Here's how the part is built. I have some questions about the finished solid (model axes, mm). Face numbers are marked on the shaded views. A direction names the side the tool comes from. Coordinates: 2 decimals unless noted, no trailing zeros. Order: outer loops, then holes, each group sorted by start corner. A loop starts at its lowest first (then second) coordinate and runs counter-clockwise, first axis right, second up. Notation, with made-up numbers: (-29.5, 79) - (-4.5, 79) arc R18 ccw to (-4.5, 103) - close; hole circle Ø1 at (-23.75, 26). An arc over 180 degrees is marked (long way). Answer in a Markdown table with one row per item. Add a question column.
Item 1: Will these pins go through, and if not, where does the flat tip stop? pin 1 Ø3 at (x, z) = (-2, 8) entering from -Y; pin 2 Ø5.5 at (x, y) = (-2.5, -0.5) entering from +Z; pin 3 Ø5 at (x, z) = (-1.5, 10) entering from -Y; pin 4 Ø2 at (y, z) = (-3.5, 7.5) entering from +X.
Item 2: I want a section at C-C (z = 4.75). Please give me the cut outline in (x, y).
Item 3: If I drill on line 1 along Z through (x, y) = (-4, 2.25); line 2 along Y through (x, z) = (0, 5.5); line 3 along Z through (x, y) = (1.75, 2.25), over which ranges is the centre line in solid material (lowest first)? Write a range as from..to.
Item 4: I want a section at A-A (y = 0). Please give me the cut outline in (x, z).
Item 5: I want a section at B-B (x = 4.5). Please give me the cut outline in (y, z).
Item 6: On a 3-axis mill with a long thin cutter (end or side, diameter ignored), from which of +Z, -Z, +X, -X, +Y, -Y can I reach the whole of each face in a straight line? I mean the marked faces 1 and 2. Say none if no direction works.
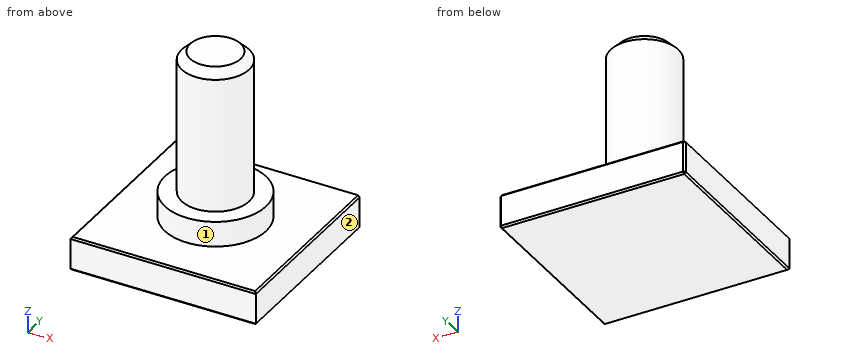
```python
from build123d import *

# Parameters (mm, degrees)
SKETCH1_W           = 11
SKETCH1_H           = 11
BOSS_EXTRUDE1_DEPTH = 2
SKETCH2_R           = 2
BOSS_EXTRUDE2_DEPTH = 10
CHAMFER1_SIZE       = 0.1
SKETCH3_R           = 3
BOSS_EXTRUDE3_DEPTH = 1.5
CHAMFER2_SIZE       = 0.5


with BuildPart() as part:
    # Sketch1 → Boss-Extrude1 (new body)
    with BuildSketch(Plane.XY):
        Rectangle(SKETCH1_W, SKETCH1_H)
    extrude(amount=BOSS_EXTRUDE1_DEPTH)

    # Sketch2 → Boss-Extrude2 (add)
    with BuildSketch(Plane.XY.offset(2)):
        Circle(SKETCH2_R)
    extrude(amount=BOSS_EXTRUDE2_DEPTH)

    # Chamfer1
    chamfer1_edges = [part.edges().sort_by_distance(p)[0] for p in [
        (-5.5, 0, 2),
        (0, -5.5, 2),
        (5.5, 0, 2),
        (0, -5.5, 0),
        (-5.5, 0, 0),
        (0, 5.5, 0),
        (5.5, 0, 0),
        (0, 5.5, 2),
        (-5.5, 5.5, 1),
        (5.5, 5.5, 1),
    ]]
    chamfer(chamfer1_edges, length=CHAMFER1_SIZE)

    # Sketch3 → Boss-Extrude3 (add)
    with BuildSketch(Plane.XY.offset(2)):
        Circle(SKETCH3_R)
    extrude(amount=BOSS_EXTRUDE3_DEPTH)

    # Chamfer2
    chamfer2_edges = [part.edges().sort_by_distance(p)[0] for p in [
        (-2, 0, 12),
    ]]
    chamfer(chamfer2_edges, length=CHAMFER2_SIZE)


solid = part.part
```
Values follow:
| question | item | result |
|---|---|---|
| 1 | pin 1 | stops at y = -1.94 |
| 1 | pin 2 | stops at z = 12 |
| 1 | pin 3 | stops at y = -2 |
| 1 | pin 4 | passes through |
| 2 | outline | circle Ø4 at (0, 0) |
| 3 | line 1 | z = 0..2 |
| 3 | line 2 | y = -2..2 |
| 3 | line 3 | z = 0..3.5 |
| 4 | outline | (-5.5, 0.1) - (-5.4, 0) - (5.4, 0) - (5.5, 0.1) - (5.5, 1.9) - (5.4, 2) - (3, 2) - (3, 3.5) - (2, 3.5) - (2, 11.5) - (1.5, 12) - (-1.5, 12) - (-2, 11.5) - (-2, 3.5) - (-3, 3.5) - (-3, 2) - (-5.4, 2) - (-5.5, 1.9) - close |
| 5 | outline | (-5.5, 0.1) - (-5.4, 0) - (5.4, 0) - (5.5, 0.1) - (5.5, 1.9) - (5.4, 2) - (-5.4, 2) - (-5.5, 1.9) - close |
| 6 | face 1 | +Z |
| 6 | face 2 | +Z, -Z, +X, +Y, -Y |
